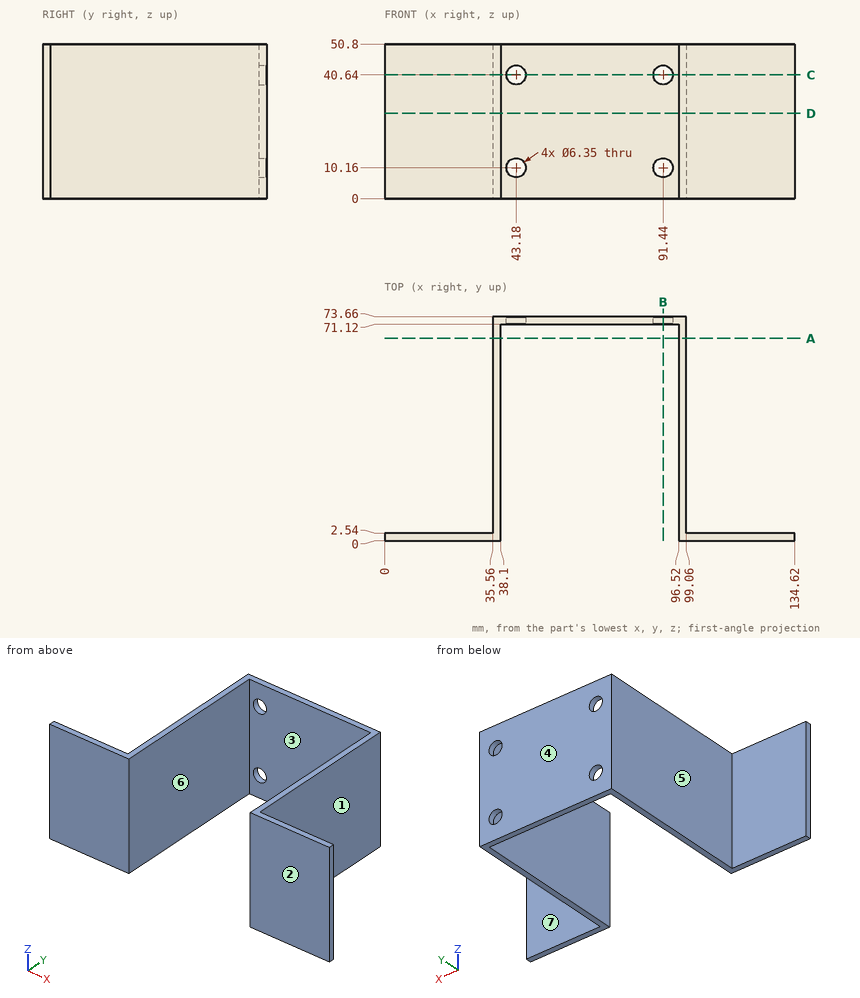
Check sheet for the drawn part. Datum: minimum x, y, z corner. Units: mm. A direction names the side the tool comes from. Round coordinates to 2 decimals unless told otherwise and drop trailing zeros. Loops run counter-clockwise (first coordinate to the right, second up) from the corner with the lowest first, then second, coordinate; pieces in that order, holes last. Notation, with made-up numbers: M -32,35.25 L -23,35.25 A20 cw -23,39.25 Z; hole C 54,5 d3. An arc over 180 degrees is marked long. One line per question, with ' | ' between items. Start each with the question number.
Item 1: Gauge pin test, flat ends, axial feed: pin 1 Ø3 at (x, z) = (109, 10) entering from -Y; pin 2 Ø1.5 at (y, z) = (25, 25.5) entering from -X; pin 3 Ø1 at (x, z) = (17, 41.5) entering from +Y; pin 4 Ø4 at (x, z) = (43.18, 10.16) entering from +Y. Record the tip position at first contact, or that the pin passes through.
Item 2: Section check B-B (x = 91.44). Record the boundary of the cut face in (y, z) (3 decimals), and give its area (3 significant figures).
Item 3: Section check D-D (z = 28). Record the boundary of the cut face in (x, y).
Item 4: Scan lines: probe 1 along Z at (x, y) = (43.18, 72.3) (3 decimals); probe 2 along X at (y, z) = (72.7, 10.16) (3 decimals); probe 3 along X at (y, z) = (15, 4). Record each from-to range of solid material in increasing order.
Item 5: Section check C-C (z = 40.64). Record the boundary of the cut face in (x, y) (3 decimals), and give its area (3 significant figures).
Item 6: Release check for a two-part mould opening along X. For the marked faces 1, 2 and 3 record: released by +X, released by -X, zero draft, split by the parting line, or undercut.
Item 7: Set-up check for the marked faces 4, 5, 6 and 7: record each of +Z, -Z, +X, -X, +Y, -Y from which the full face is reachable in a straight line by a thin tool's end or side.
Item 8: Section check A-A (y = 66.5). Record the boundary of the cut face in (x, z), and give its area (3 significant figures).
Worked out:
1) pin 1: y = 0 | pin 2: x = 35.56 | pin 3: y = 2.54 | pin 4: through
2) outline: M 71.12,0 L 73.66,0 L 73.66,6.985 L 71.12,6.985 Z; M 71.12,13.335 L 73.66,13.335 L 73.66,37.465 L 71.12,37.465 Z; M 71.12,43.815 L 73.66,43.815 L 73.66,50.8 L 71.12,50.8 Z | area: 96.8 mm^2
3) outline: M 0,0 L 38.1,0 L 38.1,71.12 L 96.52,71.12 L 96.52,0 L 134.62,0 L 134.62,2.54 L 99.06,2.54 L 99.06,73.66 L 35.56,73.66 L 35.56,2.54 L 0,2.54 Z
4) probe 1: 0 to 6.985, 13.335 to 37.465, 43.815 to 50.8 | probe 2: 35.56 to 40.005, 46.355 to 88.265, 94.615 to 99.06 | probe 3: 35.56 to 38.1, 96.52 to 99.06
5) outline: M 0,0 L 38.1,0 L 38.1,71.12 L 40.005,71.12 L 40.005,73.66 L 35.56,73.66 L 35.56,2.54 L 0,2.54 Z; M 46.355,71.12 L 88.265,71.12 L 88.265,73.66 L 46.355,73.66 Z; M 94.615,71.12 L 96.52,71.12 L 96.52,0 L 134.62,0 L 134.62,2.54 L 99.06,2.54 L 99.06,73.66 L 94.615,73.66 Z | area: 671 mm^2
6) face 1: released by +X | face 2: zero draft | face 3: undercut
7) face 4: +Z, -Z, +X, -X, +Y | face 5: +Z, -Z, -X, +Y | face 6: +Z, -Z, -Y | face 7: +Z, -Z, +X, +Y
8) outline: M 35.56,0 L 38.1,0 L 38.1,50.8 L 35.56,50.8 Z; M 96.52,0 L 99.06,0 L 99.06,50.8 L 96.52,50.8 Z | area: 258 mm^2
